Design review of the part shown in the three views and the two pictorial views. Dimensions are in mm from the part's minimum x, y and z. A direction names the side the tool comes from. Give positions to 0.01 mm unless a question says otherwise; leave off trailing zeros. Order: outer loops, then holes, each group sorted by start corner. A loop starts at its lowest first (then second) coordinate and runs counter-clockwise, first axis right, second up. Notation, with made-up numbers: (78.5, 68) -> (103.5, 68) arc R10 cw to (103.5, 74) -> close; hole circle Ø7 at (-20, 4.5). An arc over 180 degrees is marked (long way). Use one line per item in the form item = value.
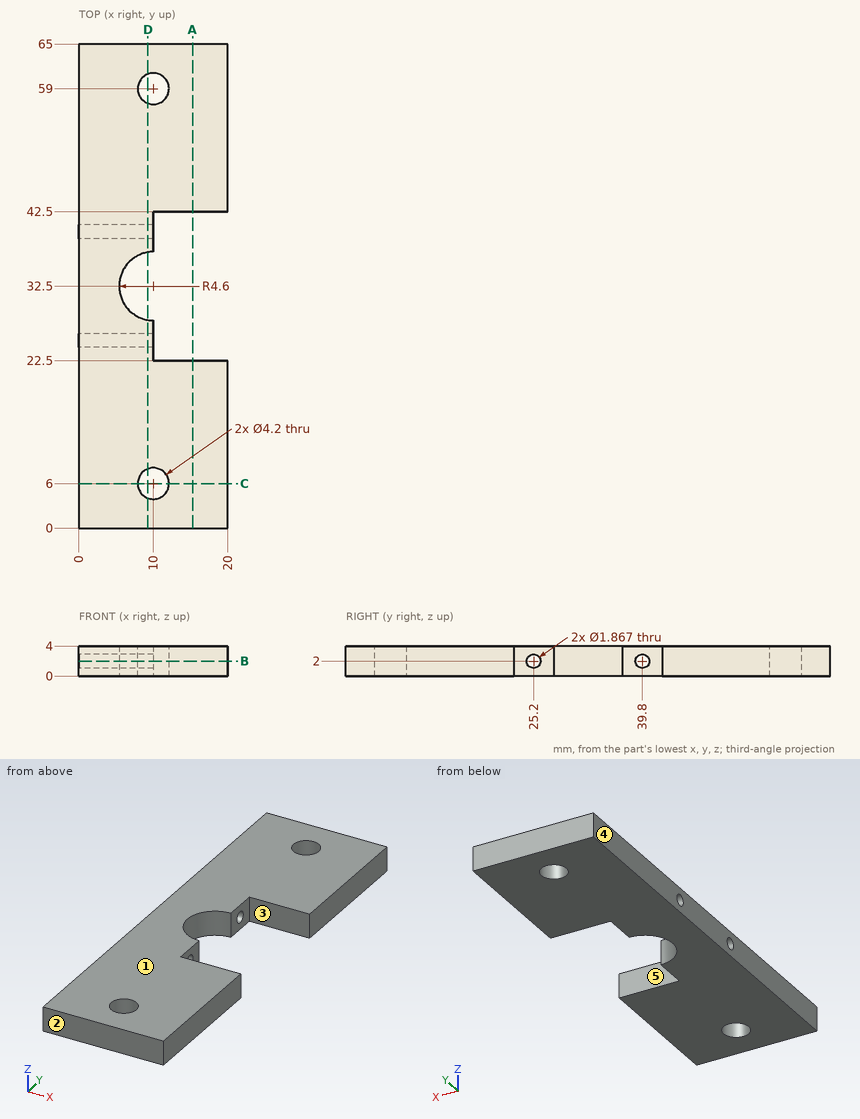
1. For pin 1 Ø2 at (y, z) = (25, 2.5) entering from +X; pin 2 Ø1 at (y, z) = (25, 2) entering from -X; pin 3 Ø2 at (y, z) = (37.5, 0.5) entering from -X, all flat-tipped, find the tip position at first contact; note any pin that passes through.
Values:
pin_1 = 10
pin_2 = through
pin_3 = 0
2. Add section B-B on z = 2. Give the boundary of the cut face in (x, y).
Values:
outline = (0, 0) -> (20, 0) -> (20, 22.5) -> (10, 22.5) -> (10, 24.27) -> (0, 24.27) -> close; (0, 26.13) -> (10, 26.13) -> (10, 27.9) arc R4.6 cw to (10, 37.1) -> (10, 38.87) -> (0, 38.87) -> close; (0, 40.73) -> (10, 40.73) -> (10, 42.5) -> (20, 42.5) -> (20, 65) -> (0, 65) -> close; hole circle Ø4.2 at (10, 6); hole circle Ø4.2 at (10, 59)
3. Add section C-C on y = 6. Give the boundary of the cut face in (x, z), then the cut area to 3 significant figures.
Values:
outline = (0, 0) -> (7.9, 0) -> (7.9, 4) -> (0, 4) -> close; (12.1, 0) -> (20, 0) -> (20, 4) -> (12.1, 4) -> close
area = 63.2 mm^2
4. Add section D-D on x = 9.25. Give the boundary of the cut face in (y, z), then the cut area to 3 significant figures.
Values:
outline = (0, 0) -> (4.04, 0) -> (4.04, 4) -> (0, 4) -> close; (7.96, 0) -> (27.96, 0) -> (27.96, 4) -> (7.96, 4) -> close; (37.04, 0) -> (57.04, 0) -> (57.04, 4) -> (37.04, 4) -> close; (60.96, 0) -> (65, 0) -> (65, 4) -> (60.96, 4) -> close; hole circle Ø1.87 at (25.2, 2); hole circle Ø1.87 at (39.8, 2)
area = 187 mm^2
5. For L1, parallel to Y at x = 4.25, z = 2; L2, parallel to X at y = 6, z = 1.8; L3, parallel to Y at x = 3, z = 2.7, list the stretches that pass through material, from the lowest coordinate up.
Values:
L1 = 0 to 24.27, 26.13 to 38.87, 40.73 to 65
L2 = 0 to 7.9, 12.1 to 20
L3 = 0 to 24.58, 25.82 to 39.18, 40.42 to 65
6. Tool access review of the marked faces 4 and 5: name each direction out of +Z, -Z, +X, -X, +Y, -Y from which nothing blocks a thin tool from reaching the whole face with its end or side.
Values:
face_4 = +Z, -Z, -X, +Y, -Y
face_5 = +Z, -Z, +X
7. Add section A-A on x = 15.25. Give the boundary of the cut face in (y, z), then the cut area to 3 significant figures.
Values:
outline = (0, 0) -> (22.5, 0) -> (22.5, 4) -> (0, 4) -> close; (42.5, 0) -> (65, 0) -> (65, 4) -> (42.5, 4) -> close
area = 180 mm^2
8. The part is to be moulded in two halves that separate along Y. For the marked faces 1, 2 and 3, say which applies: +Y half, -Y half, draft (parallel to the pull), parting line (faces both ways), or undercut.
Values:
face_1 = draft
face_2 = -Y half
face_3 = undercut
